from build123d import *

# Parameters (mm, degrees)
F2_DEPTH = 12.7
F1_W     = 12.8612825647
F1_H     = 50.9009920061
F3_DEPTH = 50.8
F4_R     = 6.5875733698
F5_DEPTH = 41.656


with BuildPart() as f2:
    # F0 (on Top) → F2 (new body)
    with BuildSketch(Plane.XY):
        Polygon((0, 25.4809688777), (0, 0), (0, -25.5783628672), (50.953771919, -25.5783628672), (50.953771919, 25.4809688777), align=None)
    extrude(amount=F2_DEPTH)

    # F1 (on Top) → F3 (join)
    with BuildSketch(Plane.XY):
        with Locations((-6.4306412823, -0.0304728746)):
            Rectangle(F1_W, F1_H)
    extrude(amount=F3_DEPTH)

    # F4 (on face) → F5 (cut)
    with BuildSketch(Plane.YZ):
        with Locations((0, 32.6068140566)):
            Circle(F4_R)
    extrude(amount=-F5_DEPTH, mode=Mode.SUBTRACT)


solid = f2.part
Geometry: final body of the model. Coordinates: model frame, mm. A direction names the side the tool comes from. Give positions to 0.01 mm unless a question says otherwise; leave off trailing zeros. Loops run counter-clockwise (first coordinate to the right, second up) from the corner with the lowest first, then second, coordinate; pieces in that order, holes last. Notation, with made-up numbers: M 60.25,-34.75 L 115.25,-34.75 A20 cw 115.25,-21.75 Z; hole C 88,-40 d9. An arc over 180 degrees is marked long. Put each result on its own line as item: value.
1) Reachability of faces 4 (the flat face through (19, 0, 0)), 5 (the flat face through (0, -6, 27)), 6 (the flat face through (-7, -25.481, 25)) from +Z, -Z, +X, -X, +Y, -Y: full face, straight path, thin tool, end or side. Return the list, or none.
Computed values:
face 4: -Z, +X, -X, +Y, -Y
face 5: +Z, +X, +Y, -Y
face 6: +Z, -Z, -X, -Y
2) Mould query, pull axis Y, two halves, no side actions, for faces 1 (the cylindrical face through (-6.341, -1.428, 26.176)), 2 (the flat face through (-7, 25.42, 25)), 3 (the flat face through (25, -25.578, 6)). Classes: released by +Y, released by -Y, zero draft, split by the parting line, or undercut.
Computed values:
face 1: undercut
face 2: released by +Y
face 3: released by -Y
3) Cut plane B-B, the plane z = 30.5. Return the cut outline in (x, y).
Computed values:
outline: M -12.86,-25.48 L 0,-25.48 L 0,-6.24 L -12.86,-6.24 Z; M -12.86,6.24 L 0,6.24 L 0,25.42 L -12.86,25.42 Z
4) First-contact query: P1, Ø8, axis at x = 32.5, y = -17, coming from the +Z side; P2, Ø6.5, axis at x = -9.5, z = 36.5, coming from the +Y side; P3, Ø1.5, axis at y = -19, z = 20, coming from the +X side. Flat tips, straight axial feed; report the tip coordinate or a pass-through.
Computed values:
P1: stops at z = 12.7
P2: stops at y = 25.42
P3: stops at x = 0
5) Cut plane D-D, the plane z = 46.5. Return the cut outline in (x, y).
Computed values:
outline: M -12.86,-25.48 L 0,-25.48 L 0,25.42 L -12.86,25.42 Z
6) Cut plane C-C, the plane y = -14. Return the cut outline in (x, z), plus the area to 3 significant figures.
Computed values:
outline: M -12.86,0 L 50.95,0 L 50.95,12.7 L 0,12.7 L 0,50.8 L -12.86,50.8 Z
area: 1,300 mm^2
7) Cut plane A-A, the plane y = 0. Return the cut outline in (x, z).
Computed values:
outline: M -12.86,0 L 50.95,0 L 50.95,12.7 L 0,12.7 L 0,26.02 L -12.86,26.02 Z; M -12.86,39.19 L 0,39.19 L 0,50.8 L -12.86,50.8 Z
8) Material intervals for L1, parallel to Z at x = -9.5, y = 0; L2, parallel to Z at x = 38.5, y = -6.5; L3, parallel to X at y = 20.5, z = 34, sorted ascending. Write a range as from..to.
Computed values:
L1: z = 0..26.02, 39.19..50.8
L2: z = 0..12.7
L3: x = -12.86..0
